Geometry: see drawing. Coordinates: mm, zero at the bounding-box minimum. Coordinates: 2 decimals unless noted, no trailing zeros. Loops run counter-clockwise (first coordinate to the right, second up) from the corner with the lowest first, then second, coordinate; pieces in that order, holes last. Notation, with made-up numbers: (-34.5, -26) -> (23.5, -26) arc R8 cw to (23.5, -15) -> close; hole circle Ø3 at (-36.5, 18.25). An arc over 180 degrees is marked (long way). One line per item, written item: value. Start each with the question number.
Item 1: Mould query, pull axis X, two halves, no side actions, for the marked faces 1 and 2. Classes: +X half, -X half, draft (parallel to the pull), parting line (faces both ways), or undercut.
Item 2: Section query D-D on y = 1.75. Return loops of the section in (x, z), then the cut area to 3 significant figures.
Item 3: Section query A-A on z = 55. Return loops of the section in (x, y).
Item 4: Contact query for flat-ended pins moving along their axis: pin 1 Ø2.5 at (y, z) = (2.5, 26.5) entering from -X; pin 2 Ø1.5 at (y, z) = (3, 24.5) entering from +X; pin 3 Ø2.5 at (x, y) = (8, 2) entering from -Z; pin 4 Ø3 at (x, z) = (10, 55) entering from -Y. Output: stop coordinate, or through.
Item 5: Section query C-C on z = 11. Return loops of the section in (x, y), then the cut area to 3 significant figures.
Item 6: Section query B-B on x = 30. Return loops of the section in (y, z).
Item 7: Ray query, probe 1 along X at (y, z) = (1.1, 55); probe 2 along X at (y, z) = (1.05, 24.5); probe 3 along Z at (x, y) = (22, 4.2). Return the intervals inside material, ascending. Write a range as from..to.
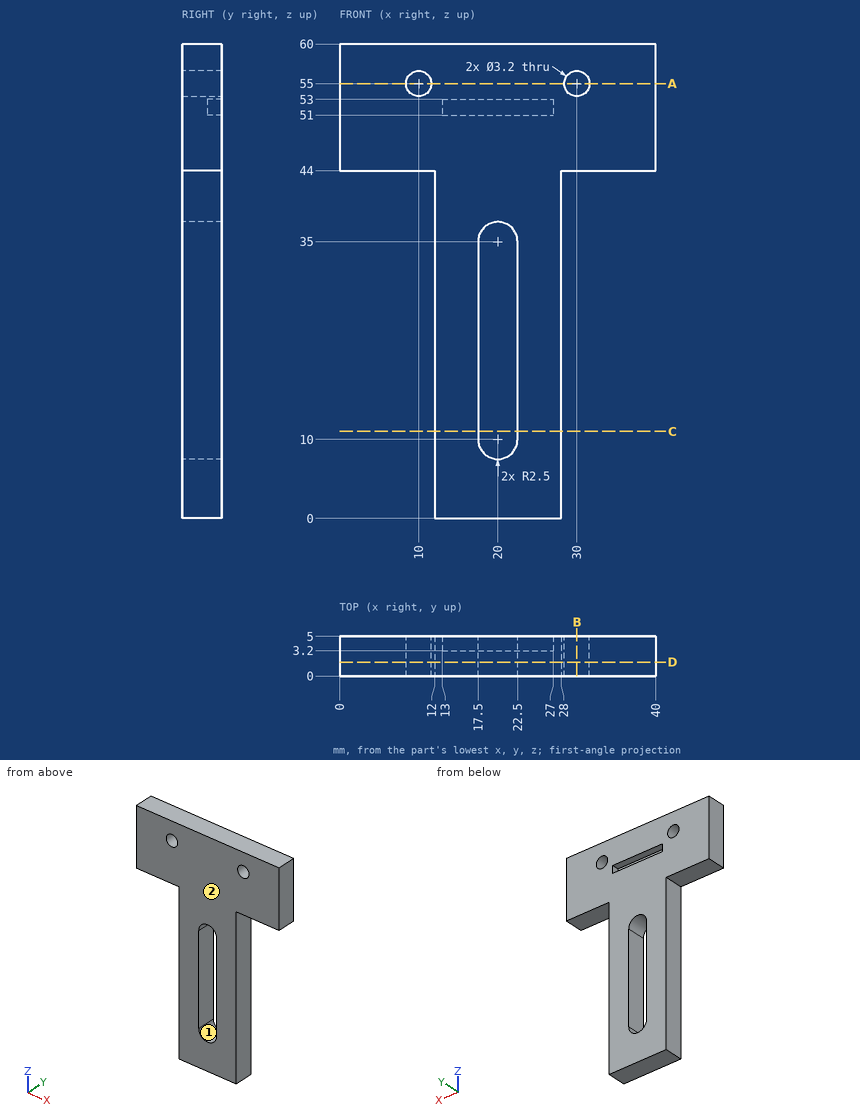
Reply:
1. face 1: undercut
1. face 2: draft
2. outline: (0, 44) -> (12, 44) -> (12, 0) -> (28, 0) -> (28, 44) -> (40, 44) -> (40, 60) -> (0, 60) -> close; hole circle Ø3.2 at (10, 55); hole (17.5, 10) arc R2.5 ccw to (22.5, 10) -> (22.5, 35) arc R2.5 ccw to (17.5, 35) -> close; hole circle Ø3.2 at (30, 55)
2. area: 1,180 mm²
3. outline: (0, 0) -> (8.4, 0) -> (8.4, 5) -> (0, 5) -> close; (11.6, 0) -> (28.4, 0) -> (28.4, 5) -> (11.6, 5) -> close; (31.6, 0) -> (40, 0) -> (40, 5) -> (31.6, 5) -> close
4. pin 1: stops at x = 12
4. pin 2: stops at x = 28
4. pin 3: stops at z = 44
4. pin 4: passes through
5. outline: (12, 0) -> (17.5, 0) -> (17.5, 5) -> (12, 5) -> close; (22.5, 0) -> (28, 0) -> (28, 5) -> (22.5, 5) -> close
5. area: 55.0 mm²
6. outline: (0, 44) -> (5, 44) -> (5, 53.4) -> (0, 53.4) -> close; (0, 56.6) -> (5, 56.6) -> (5, 60) -> (0, 60) -> close
7. probe 1: x = 0..8.4, 11.6..28.4, 31.6..40
7. probe 2: x = 12..17.5, 22.5..28
7. probe 3: z = 0..8.5, 36.5..51, 53..60
